For this review, take the finished solid that the model builds, in its own axes (mm). Give positions to 0.01 mm unless a question says otherwise; leave off trailing zeros. Order: outer loops, then holes, each group sorted by start corner. A loop starts at its lowest first (then second) coordinate and runs counter-clockwise, first axis right, second up. Notation, with made-up numbers: (56.25, 64.25) -> (77.25, 64.25) arc R14 cw to (77.25, 78.25) -> close; hole circle Ø9 at (-31, 76.25). An arc over 180 degrees is marked (long way). One line per item, written item: value. Start each with the question number.
from build123d import *

# Parameters (mm, degrees)
SKETCH_W       = 20
SKETCH_H       = 20
PAD_DEPTH      = 40
SKETCH001_R    = 1.65
HOLE_DEPTH     = 10
HOLE_TIPS_R    = 1.65
SKETCH002_R    = 1.65
HOLE001_DEPTH  = 12
HOLE001_TIPS_R = 1.65


with BuildPart() as part:
    # Sketch → Pad (new body)
    with BuildSketch(Plane.XY):
        with Locations((75, 10)):
            Rectangle(SKETCH_W, SKETCH_H)
    extrude(amount=PAD_DEPTH)

    # Sketch001 (on Face1 of Pad) → Hole (cut)
    with BuildSketch(Plane.XZ):
        with Locations((75, 30)):
            Circle(SKETCH001_R)
        with Locations((75, 10)):
            Circle(SKETCH001_R)
    extrude(amount=-HOLE_DEPTH, mode=Mode.SUBTRACT)

    # Hole tips → Hole tip 1 section 0
    with BuildSketch(Plane.XZ.offset(-10), mode=Mode.PRIVATE) as hole_tip_1_s0:
        with Locations((75, 30)):
            Circle(HOLE_TIPS_R)
    loft([hole_tip_1_s0.sketch, Vertex(75, 10.99142, 30)], mode=Mode.SUBTRACT)

    # Hole tips → Hole tip 2 section 0
    with BuildSketch(Plane.XZ.offset(-10), mode=Mode.PRIVATE) as hole_tip_2_s0:
        with Locations((75, 10)):
            Circle(HOLE_TIPS_R)
    loft([hole_tip_2_s0.sketch, Vertex(75, 10.99142, 10)], mode=Mode.SUBTRACT)

    # Sketch002 (on Face4 of Hole) → Hole001 (cut)
    with BuildSketch(Plane.XY.offset(40)):
        with Locations((70, 10)):
            Circle(SKETCH002_R)
    extrude(amount=-HOLE001_DEPTH, mode=Mode.SUBTRACT)

    # Hole001 tips → Hole001 tip 1 section 0
    with BuildSketch(Plane.XY.offset(28), mode=Mode.PRIVATE) as hole001_tip_1_s0:
        with Locations((70, 10)):
            Circle(HOLE001_TIPS_R)
    loft([hole001_tip_1_s0.sketch, Vertex(70, 10, 27.00858)], mode=Mode.SUBTRACT)


solid = part.part
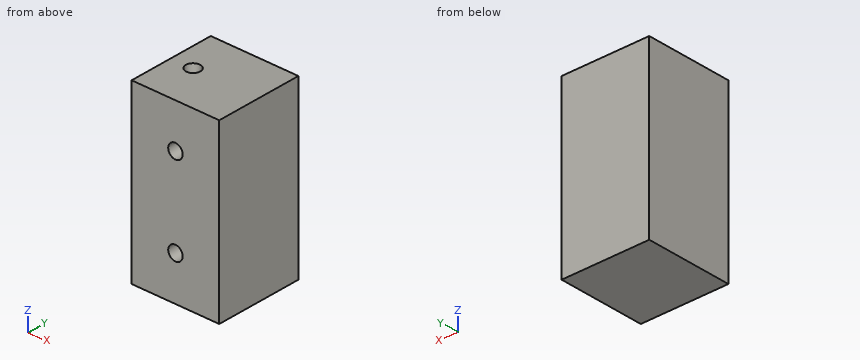
Q1. For pin 1 Ø2 at (x, y) = (70, 10) entering from +Z, flat-tipped, find the tip position at first contact; note if it passes through.
Q2. Take a section at A-A (y = 5.25). State the section outline as (x, z) points, and give its area (3 significant figures).
Q3. For line 1 along Z through (x, y) = (75, 4); line 2 along Z through (x, y) = (75.75, 1.5); line 3 along X through (y, z) = (10.25, 36), list the stretches that pass through material, from the lowest coordinate up.
Answers below:
1. pin 1: stops at z = 27.61
2. outline: (65, 0) -> (85, 0) -> (85, 40) -> (65, 40) -> close; hole circle Ø3.3 at (75, 10); hole circle Ø3.3 at (75, 30)
2. area: 783 mm²
3. line 1: z = 0 to 8.35, 11.65 to 28.35, 31.65 to 40
3. line 2: z = 0 to 8.53, 11.47 to 28.53, 31.47 to 40
3. line 3: x = 65 to 68.37, 71.63 to 85
